Can you work these out from the model? Positions are in its coordinate system, mm. Face numbers are marked on the shaded views. Coordinates: 2 decimals unless noted, no trailing zeros. Write each loop counter-clockwise with the first axis right and the second up, starting at its lowest first coordinate (ties: lowest second). Pieces come first, ordered by that corner, then holes. Notation, with made-up numbers: M 51.25,1 L 79.25,1 A31 ccw 79.25,34 Z; hole C 24.5,15 d4. An arc over 180 degrees is marked long. Answer as a JSON object with one key per item and string values. Group by question number.
Autodesk Inventor part; units mm, degrees
ref_plane "YZ Plane" through (0, 0, 0) normal (1, 0, 0) x (0, 1, 0)
ref_plane "XZ Plane" through (0, 0, 0) normal (0, 1, 0) x (-1, 0, 0)
ref_plane "XY Plane" through (0, 0, 0) normal (0, 0, 1) x (1, 0, 0)
sketch "Sketch1" plane through (0, 0, 0) normal (0, 1, 0) x (-1, 0, 0)
  circle A0 centre (0, 0) radius 1.4605
  dimension "d0" = 2.921
extrude "Extrusion1" add sketch "Sketch1" along normal blind 21.59
sketch "Sketch2" plane through (0, 21.59, 0) normal (0, 1, 0) x (1, 0, 0)
  circle A0 centre (0, 0) radius 2.54
  dimension "d3" = 5.08
extrude "Extrusion2" add sketch "Sketch2" along normal blind 3.175
sketch "Sketch3" plane through (0, 24.765, 0) normal (0, 1, 0) x (1, 0, 0)
  line L0 (0, 1.8331) -> (1.5875, 0.9165)
  line L1 (1.5875, 0.9165) -> (1.5875, -0.9165)
  line L2 (1.5875, -0.9165) -> (0, -1.8331)
  line L3 (0, -1.8331) -> (-1.5875, -0.9165)
  line L4 (-1.5875, -0.9165) -> (-1.5875, 0.9165)
  line L5 (-1.5875, 0.9165) -> (0, 1.8331)
  point P0 (0, 0)
  point P1 (0, 0)
  dimension "d6" = 3.175
extrude "Extrusion3" cut sketch "Sketch3" against normal blind 1.905
thread "Thread1"
properties part number "Tube Rack bolt" material "Steel, Galvanized"
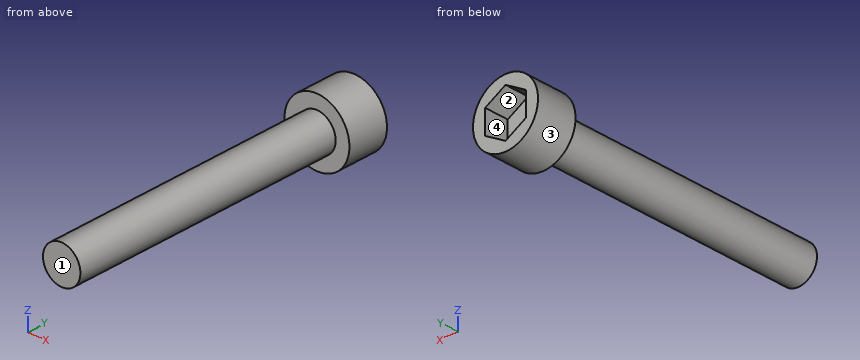
Q1. Please list where these lines run through material, in increasing order: L1, parallel to Y at x = 1.75, z = 0.65 (3 decimals); L2, parallel to Y at x = -0.8, z = 0.1; L3, parallel to Z at x = -0.3, y = 23.5.
Q2. If we section it at A-A on y = 23.25: List the corners of the cut face in (x, z) for me, and give its area (3 significant figures).
Q3. If we section it at D-D on y = 15: List the corners of the cut face in (x, z) for me.
Q4. Will these pins go through, and if not, where does the flat tip stop? pin 1 (1.6 mm diameter, centred on x = -0.5, z = 0, fed in from +Y); pin 2 (3 mm diameter, centred on x = 0, y = 11.5, fed in from +Z); pin 3 (1.5 mm diameter, centred on x = -1, y = 9, fed in from -Z).
Q5. We'd pull the mould along X, two halves only. Please class the marked faces 1, 2, 3 and 4: pulls with the +X half, pulls with the -X half, needs draft (parallel to the pull), parting line crosses it, or undercut.
Q6. If we section it at C-C on x = -0.9: List the corners of the cut face in (y, z) for me (3 decimals).
Q7. If we section it at B-B on z = 0: List the corners of the cut face in (x, y) for me (1 decimal), and give its area (3 significant figures).
Reply:
{
 "1": {"L1": "21.59 to 24.765", "L2": "0 to 22.86", "L3": "-2.52 to -1.66, 1.66 to 2.52"},
 "2": {"outline": "C 0,0 d5.08; hole M -1.59,-0.92 L 0,-1.83 L 1.59,-0.92 L 1.59,0.92 L 0,1.83 L -1.59,0.92 Z", "area": "11.5 mm^2"},
 "3": {"outline": "C 0,0 d2.92"},
 "4": {"pin 1": "y = 22.86", "pin 2": "z = 1.46", "pin 3": "z = -1.44"},
 "5": {"face 1": "needs draft", "face 2": "undercut", "face 3": "parting line crosses it", "face 4": "undercut"},
 "6": {"outline": "M 0,-1.15 L 21.59,-1.15 L 21.59,-2.375 L 24.765,-2.375 L 24.765,-1.313 L 22.86,-1.313 L 22.86,1.313 L 24.765,1.313 L 24.765,2.375 L 21.59,2.375 L 21.59,1.15 L 0,1.15 Z"},
 "7": {"outline": "M -2.5,21.6 L -1.5,21.6 L -1.5,0 L 1.5,0 L 1.5,21.6 L 2.5,21.6 L 2.5,24.8 L 1.6,24.8 L 1.6,22.9 L -1.6,22.9 L -1.6,24.8 L -2.5,24.8 Z", "area": "73.1 mm^2"}
}
